```python
from build123d import *

# Parameters (mm, degrees)
SKETCH1_W           = 30
SKETCH1_H           = 30
BOSS_EXTRUDE1_DEPTH = 150
SKETCH2_R           = 7.5
CUT_EXTRUDE1_DEPTH  = 150


with BuildPart() as part:
    # Sketch1 → Boss-Extrude1 (new body)
    with BuildSketch(Plane.XY):
        Rectangle(SKETCH1_W, SKETCH1_H)
    extrude(amount=BOSS_EXTRUDE1_DEPTH)

    # Sketch2 → Cut-Extrude1 (cut)
    with BuildSketch(Plane.XZ.offset(15)):
        with Locations(Location((0, 30, 0), (0, 0, 270))):
            Circle(SKETCH2_R)
    extrude(amount=-CUT_EXTRUDE1_DEPTH, mode=Mode.SUBTRACT)


solid = part.part
```
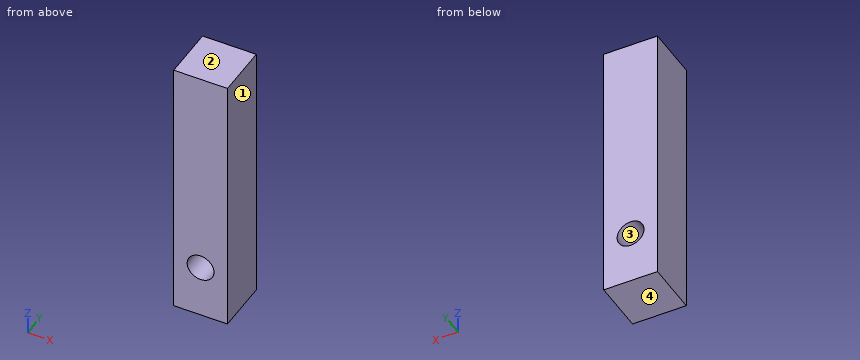
Geometry check sheet. Reference: the model listing, model coordinates, mm. Face numbers are marked on the shaded views. Give positions to 0.01 mm unless a question says otherwise; leave off trailing zeros. Order: outer loops, then holes, each group sorted by start corner. A loop starts at its lowest first (then second) coordinate and runs counter-clockwise, first axis right, second up.
1. Section check B-B, the plane x = 0. Enter the section's corners in (y, z), and give its area (3 significant figures).
2. Section check A-A, the plane z = 30. Enter the section's corners in (x, y).
3. Release check for a two-part mould opening along Z. For the marked faces 1, 2, 3 and 4 record: pulls with the +Z half, pulls with the -Z half, needs draft (parallel to the pull), parting line crosses it, or undercut.
4. Section check C-C, the plane y = -8.5. Enter the section's corners in (x, z).
5. Thickness scan on L1, parallel to X at y = 7.25, z = 30; L2, parallel to Z at x = -1.75, y = -2.75; L3, parallel to Z at x = 0.75, y = -12.25. Record the ranges inside material, lowest first.
Values follow:
1. outline: (-15, 0) - (15, 0) - (15, 22.5) - (-15, 22.5) - close; (-15, 37.5) - (15, 37.5) - (15, 150) - (-15, 150) - close
1. area: 4,050 mm2
2. outline: (-15, -15) - (-7.5, -15) - (-7.5, 15) - (-15, 15) - close; (7.5, -15) - (15, -15) - (15, 15) - (7.5, 15) - close
3. face 1: needs draft
3. face 2: pulls with the +Z half
3. face 3: undercut
3. face 4: pulls with the -Z half
4. outline: (-15, 0) - (15, 0) - (15, 150) - (-15, 150) - close; hole circle Ø15 at (0, 30)
5. L1: x = -15 to -7.5, 7.5 to 15
5. L2: z = 0 to 22.71, 37.29 to 150
5. L3: z = 0 to 22.54, 37.46 to 150
